Part model, mm, in its own coordinate system. A direction names the side the tool comes from. Give positions to 0.01 mm unless a question says otherwise; leave off trailing zeros. Order: outer loops, then holes, each group sorted by start corner. A loop starts at its lowest first (then second) coordinate and runs counter-clockwise, first axis right, second up. Notation, with made-up numbers: (-34.75, 4) - (-2.75, 4) arc R28 ccw to (-2.75, 36) - close; hole circle Ø5 at (-3.75, 18). An arc over 180 degrees is marked (long way). Use one line per item in the form item = value. Start each with the question number.
1. Band-saw the part on C-C, the plane z = 10. List the corners of the cut face in (x, y).
2. Pin check, flat tips, straight feed: P1, Ø1, axis at x = -8.5, z = 12.5, coming from the +Y side; P2, Ø1, axis at x = -12, y = 3.5, coming from the +Z side; P3, Ø3, axis at y = 6.5, z = -12, coming from the -X side. Stop position of each tip, or through.
3. Band-saw the part on A-A, the plane y = 5.5. List the corners of the cut face in (x, z), plus the area to 3 significant figures.
4. Band-saw the part on B-B, the plane x = -10. List the corners of the cut face in (y, z), plus the area to 3 significant figures.
5. Drill centre lines: line 1 (Y direction, x = -1, z = 6); line 2 (X direction, y = 1.5, z = -10.5); line 3 (Y direction, x = -15.5, z = 3). Where is each one in solid material? Low to high.
6. Tool access for faces 5 (the face through (6.24, 1.74, 7.33)), 6 (the face through (-18.361, 6.226, 0.064)), 7 (the face through (-9.992, 1.74, 9.867)): list every direction of +Z, -Z, +X, -X, +Y, -Y with a clear straight run to the whole face (end or side of a thin tool).
7. Pull direction Z, two halves, no side cores. Call faces 1 (the face through (-15.891, 5.24, -0.255)), 2 (the face through (2.807, 1.76, -5.617)), 3 (the face through (4, 1, -0.855)), 4 (the face through (-11, 0, 8)): +Z half, -Z half, draft (parallel to the pull), parting line (faces both ways), or undercut.
from build123d import *

# Parameters (mm, degrees)
BOSS_EXTRUDE2_DEPTH     = 4.5
CUT_EXTRUDE1_DEPTH      = 3
BOSS_EXTRUDE3_DEPTH     = 3.5
CUT_EXTRUDE2_DEPTH      = 15.5
CUT_EXTRUDE2_DEPTH_BACK = 34.485281374
CUT_EXTRUDE5_DEPTH      = 34.485281374
SKETCH10_W              = 4
SKETCH10_H              = 1.5
CUT_EXTRUDE6_DEPTH      = 2
SKETCH11_W              = 4
SKETCH11_H              = 1.5
CUT_EXTRUDE7_DEPTH      = 2
SKETCH12_W              = 4
SKETCH12_H              = 1.5
CUT_EXTRUDE8_DEPTH      = 2
SKETCH13_W              = 4
SKETCH13_H              = 1.5
CUT_EXTRUDE9_DEPTH      = 2


with BuildPart() as part:
    # Sketch2 → Boss-Extrude2 (new body)
    with BuildSketch(Plane(origin=(0, 0, 0), x_dir=(1, 0, 0), z_dir=(0, 1, 0))):
        Polygon((-4.567545122, 15.820593449), (13.110124407, -1.85707608), (-3.14292392, -18.110124407), (-20.820593449, -0.432454878), align=None)
    extrude(amount=BOSS_EXTRUDE2_DEPTH)

    # Sketch4 → Cut-Extrude1 (cut)
    with BuildSketch(Plane(origin=(0, 0, 0), x_dir=(1, 0, 0), z_dir=(0, 1, 0))):
        Polygon((-18.008282848, -3.244765479), (-5.905234521, -3.244765479), (-5.905234521, -15.347813806), (-3.14292392, -18.110124407), (-1.805234521, -16.772435009), (-1.805234521, -3.244765479), (11.722435009, -3.244765479), (13.110124407, -1.85707608), (10.397813806, 0.855234521), (-1.832165216, 0.855234521), (-1.99606638, 13.249114707), (-4.567545122, 15.820593449), (-5.905234521, 14.482904051), (-5.905234521, 0.855234521), (-19.532904051, 0.855234521), (-20.820593449, -0.432454878), align=None)
    extrude(amount=CUT_EXTRUDE1_DEPTH, mode=Mode.SUBTRACT)

    # Sketch5 → Boss-Extrude3 (add)
    with BuildSketch(Plane(origin=(0, 4.5, 0), x_dir=(1, 0, 0), z_dir=(0, 1, 0))):
        Polygon((8.86748372, -6.099716767), (11.695910845, -3.271289643), (9.574590502, -1.149969299), (6.746163377, -3.978396424), align=None)
        Polygon((-6.688865466, 9.456632419), (-3.860438341, 12.285059543), (-5.981758685, 14.406379887), (-8.810185809, 11.577952762), align=None)
        Polygon((-17.285059543, -1.139561659), (-14.456632419, 1.688865466), (-16.577952762, 3.810185809), (-19.406379887, 0.981758685), align=None)
        Polygon((-1.728710357, -16.695910845), (1.099716767, -13.86748372), (-1.021603576, -11.746163377), (-3.850030701, -14.574590502), align=None)
    extrude(amount=BOSS_EXTRUDE3_DEPTH)

    # Sketch6 → Cut-Extrude2 (cut, two sides)
    with BuildSketch(Plane(origin=(4.212310601, 0, -4.212310601), x_dir=(-0.707106781, 0, -0.707106781), z_dir=(0.707106781, 0, -0.707106781))) as cut_extrude2_sk:
        with BuildLine():
            Line((-7.58340896, 6), (-7.58340896, 7.2))
            ThreePointArc((-7.58340896, 7.2), (-8.18340896, 6.6), (-7.58340896, 6))
        make_face()
    extrude(amount=CUT_EXTRUDE2_DEPTH, mode=Mode.SUBTRACT)
    extrude(cut_extrude2_sk.sketch, amount=-CUT_EXTRUDE2_DEPTH_BACK, mode=Mode.SUBTRACT)

    # Sketch7 → Cut-Extrude5 (cut, through all)
    with BuildSketch(Plane(origin=(4.212310601, 0, -4.212310601), x_dir=(-0.707106781, 0, -0.707106781), z_dir=(0.707106781, 0, -0.707106781))):
        with BuildLine():
            Line((11.41659104, 7.2), (11.41659104, 6))
            ThreePointArc((11.41659104, 6), (12.01659104, 6.6), (11.41659104, 7.2))
        make_face()
    extrude(amount=-CUT_EXTRUDE5_DEPTH, mode=Mode.SUBTRACT)

    # Sketch10 → Cut-Extrude6 (cut)
    with BuildSketch(Plane(origin=(5.626524164, 0, -5.626524164), x_dir=(-0.707106781, 0, -0.707106781), z_dir=(0.707106781, 0, -0.707106781))):
        with Locations((2.014970927, 1.75)):
            Rectangle(SKETCH10_W, SKETCH10_H)
    extrude(amount=-CUT_EXTRUDE6_DEPTH, mode=Mode.SUBTRACT)

    # Sketch11 → Cut-Extrude7 (cut)
    with BuildSketch(Plane(origin=(-10.626524164, 0, 10.626524164), x_dir=(0.707106781, 0, 0.707106781), z_dir=(-0.707106781, 0, 0.707106781))):
        with Locations((-2.088088155, 1.75)):
            Rectangle(SKETCH11_W, SKETCH11_H)
    extrude(amount=-CUT_EXTRUDE7_DEPTH, mode=Mode.SUBTRACT)

    # Sketch12 → Cut-Extrude8 (cut)
    with BuildSketch(Plane(origin=(7.483600244, 0, 7.483600244), x_dir=(0.707106781, 0, -0.707106781), z_dir=(0.707106781, 0, 0.707106781))):
        with Locations((-2.770382387, 1.75)):
            Rectangle(SKETCH12_W, SKETCH12_H)
    extrude(amount=-CUT_EXTRUDE8_DEPTH, mode=Mode.SUBTRACT)

    # Sketch13 → Cut-Extrude9 (cut)
    with BuildSketch(Plane(origin=(-10.194069286, 0, -10.194069286), x_dir=(-0.707106781, 0, 0.707106781), z_dir=(-0.707106781, 0, -0.707106781))):
        with Locations((4.442106781, 1.75)):
            Rectangle(SKETCH13_W, SKETCH13_H)
    extrude(amount=-CUT_EXTRUDE9_DEPTH, mode=Mode.SUBTRACT)


solid = part.part
From the geometry:
q1.outline = (-11.25, 0) - (-5.91, 0) - (-5.91, 3) - (-1.81, 3) - (-1.81, 0) - (4.97, 0) - (4.97, 1) - (3.25, 1) - (3.25, 2.5) - (4.97, 2.5) - (4.97, 4.5) - (-11.25, 4.5) - (-11.25, 2.5) - (-10.12, 2.5) - (-10.12, 1) - (-11.25, 1) - close
q2.P1 = 4.5
q2.P2 = 9.75
q2.P3 = -8.81
q3.outline = (-19.41, -0.98) - (-16.58, -3.81) - (-14.46, -1.69) - (-17.29, 1.14) - close; (-8.81, -11.58) - (-5.98, -14.41) - (-3.86, -12.29) - (-6.69, -9.46) - close; (-3.85, 14.57) - (-1.02, 11.75) - (1.1, 13.87) - (-1.73, 16.7) - close; (6.75, 3.98) - (9.57, 1.15) - (11.7, 3.27) - (8.87, 6.1) - close
q3.area = 48.0 mm²
q4.outline = (0, -10.39) - (4.5, -10.39) - (4.5, 11.25) - (0, 11.25) - (0, 3.24) - (3, 3.24) - (3, -0.86) - (0, -0.86) - close; hole (1, 8.42) - (2.5, 8.42) - (2.5, 9.88) - (1, 9.88) - close
q4.area = 82.9 mm²
q5.line_1 = 0 to 4.5
q5.line_2 = -9.89 to -5.91, -1.96 to 0.75
q5.line_3 = 3 to 4.5
q6.face_5 = +Z
q6.face_6 = +Z, -X, +Y
q6.face_7 = -X
q7.face_1 = +Z half
q7.face_2 = undercut
q7.face_3 = undercut
q7.face_4 = draft
